```python
from build123d import *

# Parameters (mm, degrees)
F0_R     = 3.34
F1_DEPTH = 7
F3_DEPTH = 9
F4_DEPTH = 9.001
F5_R     = 1.3
F6_W     = 3.9447422773
F6_H     = 0.2829339355
F6_W_2   = 4.4
F6_H_2   = 6.4
F7_DEPTH = 0.5


# Not quite as in the source:
# - a feature names something its author has since deleted; it is built from what else it names


with BuildPart() as f1:
    # F0 (on Right) → F1 (new body)
    with BuildSketch(Plane.YZ):
        with BuildLine():
            Line((4.5, -14.3079506601), (4.5, 14.3079506601))
            Line((4.5, 14.3079506601), (-4.5, 14.3079506601))
            Line((-4.5, 14.3079506601), (-4.5, -14.3079506601))
            ThreePointArc((-4.5, -14.3079506601), (0, -18.8079506601), (4.5, -14.3079506601))
        make_face()
        with Locations((0, -14.3079506601)):
            Circle(F0_R, mode=Mode.SUBTRACT)
    extrude(amount=F1_DEPTH)

    # F2 (on face) → F3 (join)
    with BuildSketch(Plane.XZ.offset(4.5)):
        Polygon((0, 4.22267057), (0, 14.3079506601), (-7, 14.3079506601), (-7, 0), (0, -4.4198017567), align=None)
    extrude(amount=-F3_DEPTH)

    # F2 (on face) → F4 (cut, through all)
    with BuildSketch(Plane.XZ.offset(4.5)):
        Polygon((7, 14.3079506601), (0, 14.3079506601), (0, 4.22267057), (7, 0), align=None)
    extrude(amount=-F4_DEPTH, mode=Mode.SUBTRACT)

    # F5
    f5_edges = [f1.edges().sort_by_distance(p)[0] for p in [
        (0, -4.5, 9.265311),
        (0, 0, 4.222671),
        (0, 4.5, 9.265311),
        (0, 0, 14.307951),
        (3.5, -4.5, 2.111335),
        (-3.5, -4.5, 14.307951),
        (-7, -4.5, 7.153975),
        (-3.5, -4.5, -2.209901),
        (0, -4.5, -9.363876),
        (3.5, -4.5, -14.307951),
        (7, -4.5, -7.153975),
        (0, 4.5, -9.363876),
        (-3.5, 4.5, -2.209901),
        (-7, 4.5, 7.153975),
        (-3.5, 4.5, 14.307951),
        (3.5, 4.5, 2.111335),
        (7, 4.5, -7.153975),
        (3.5, 4.5, -14.307951),
        (-7, 0, 14.307951),
        (-7, 0, 0),
        (7, 0, 0),
        (0, 0, -4.419802),
    ]]
    fillet(f5_edges, radius=F5_R)

    # F6 (on face) → F7 (cut)
    with BuildSketch(Plane.XY.offset(14.3079506601)):
        with Locations((46.5, 2.275798656)):
            Rectangle(F6_W, F6_H)
        with Locations((46.5, 0.2357986942)):
            Rectangle(F6_W, F6_H)
        with Locations((46.5, -1.8042012677)):
            Rectangle(F6_W, F6_H)
        with Locations((46.5, 0.7457986847)):
            Rectangle(F6_W, F6_H)
        with Locations((46.5, 1.2557986751)):
            Rectangle(F6_W, F6_H)
        with Locations((46.5, -2.3142012581)):
            Rectangle(F6_W, F6_H)
        with Locations((46.5, 2.7857986465)):
            Rectangle(F6_W, F6_H)
        with Locations((46.5, -0.2742012963)):
            Rectangle(F6_W, F6_H)
        with Locations((46.5, -1.2942012772)):
            Rectangle(F6_W, F6_H)
        with Locations((46.5, 1.7657986656)):
            Rectangle(F6_W, F6_H)
        with Locations((46.5, -0.7842012867)):
            Rectangle(F6_W, F6_H)
        with Locations((46.5, -2.8242012486)):
            Rectangle(F6_W, F6_H)
        with Locations((-3.5, 0)):
            Rectangle(F6_W_2, F6_H_2)
        with Locations((-3.5, -2.8242012486)):
            Rectangle(F6_W, F6_H, mode=Mode.SUBTRACT)
        with Locations((-3.5, -2.3142012581)):
            Rectangle(F6_W, F6_H, mode=Mode.SUBTRACT)
        with Locations((-3.5, -1.8042012677)):
            Rectangle(F6_W, F6_H, mode=Mode.SUBTRACT)
        with Locations((-3.5, -1.2942012772)):
            Rectangle(F6_W, F6_H, mode=Mode.SUBTRACT)
        with Locations((-3.5, -0.7842012867)):
            Rectangle(F6_W, F6_H, mode=Mode.SUBTRACT)
        with Locations((-3.5, -0.2742012963)):
            Rectangle(F6_W, F6_H, mode=Mode.SUBTRACT)
        with Locations((-3.5, 0.2357986942)):
            Rectangle(F6_W, F6_H, mode=Mode.SUBTRACT)
        with Locations((-3.5, 0.7457986847)):
            Rectangle(F6_W, F6_H, mode=Mode.SUBTRACT)
        with Locations((-3.5, 1.2557986751)):
            Rectangle(F6_W, F6_H, mode=Mode.SUBTRACT)
        with Locations((-3.5, 1.7657986656)):
            Rectangle(F6_W, F6_H, mode=Mode.SUBTRACT)
        with Locations((-3.5, 2.275798656)):
            Rectangle(F6_W, F6_H, mode=Mode.SUBTRACT)
        with Locations((-3.5, 2.7857986465)):
            Rectangle(F6_W, F6_H, mode=Mode.SUBTRACT)
    extrude(amount=-F7_DEPTH, mode=Mode.SUBTRACT)


solid = f1.part
```
Build history of the part. All positions in model axes, mm. A direction names the side the tool comes from. Round coordinates to 2 decimals unless told otherwise and drop trailing zeros. Loops run counter-clockwise (first coordinate to the right, second up) from the corner with the lowest first, then second, coordinate; pieces in that order, holes last.
Item 1: Two-plate mould, pull along Y, no slides. Class faces 1 (the face through (0, -4.5, 0)), 2 (the face through (3.451, -0.435, -10.996)), 3 (the face through (-3.251, 4.129, -1.905)), 4 (the face through (-3.541, -0.045, -2.184)): released by +Y, released by -Y, zero draft, split by the parting line, or undercut.
Item 2: Drill centre lines: line 1 along X through (y, z) = (2.75, 6); line 2 along Z through (x, y) = (6.5, -2); line 3 along X through (y, z) = (2.75, -8). Where is each one in solid material? Low to high.
Item 3: Which spindle directions (+Z, -Z, +X, -X, +Y, -Y) get a long thin tool onto all of the face, cutting with end or side? Do faces 5 (the face through (-0.37, -4.11, 8.93)), 6 (the face through (-0.39, 4.13, 8.93)). Say none if no direction does.
Item 4: Saw through at B-B (z = 6.5). List the corners of the cut face in (x, y), then the cut area to 3 significant figures.
Item 5: Pin check, flat tips, straight feed: P1, Ø0.6, axis at x = -3, z = 14, coming from the +Y side; P2, Ø4, axis at y = -1.5, z = 7, coming from the +X side; P3, Ø8, axis at x = 0.5, z = 10.5, coming from the -Y side; P4, Ø4, axis at x = -4.5, y = -2, coming from the -Z side. Stop position of each tip, or through.
Item 6: Saw through at A-A (z = -13). List the corners of the cut face in (x, y).
Worked answers:
1. face 1: released by -Y
1. face 2: undercut
1. face 3: released by +Y
1. face 4: zero draft
2. line 1: x = -7 to 0
2. line 2: z = -18.04 to -16.98, -11.63 to 0.29
2. line 3: x = 0 to 7
3. face 5: +Z, +X, -Y
3. face 6: +Z, +X, +Y
4. outline: (-7, -3.2) arc R1.3 ccw to (-5.7, -4.5) - (-1.3, -4.5) arc R1.3 ccw to (0, -3.2) - (0, 3.2) arc R1.3 ccw to (-1.3, 4.5) - (-5.7, 4.5) arc R1.3 ccw to (-7, 3.2) - close
4. area: 61.5 mm2
5. P1: stops at y = 4.3
5. P2: stops at x = 0
5. P3: stops at y = -4.5
5. P4: stops at z = -2.84
6. outline: (0, -3.2) arc R1.3 ccw to (1.3, -4.5) - (5.7, -4.5) arc R1.3 ccw to (7, -3.2) - (7, -3.07) - (0, -3.07) - close; (0, 3.07) - (7, 3.07) - (7, 3.2) arc R1.3 ccw to (5.7, 4.5) - (1.3, 4.5) arc R1.3 ccw to (0, 3.2) - close
